Geometry: final body of the model. Coordinates: model frame, mm. Face numbers are marked on the shaded views. A direction names the side the tool comes from. Round coordinates to 2 decimals unless told otherwise and drop trailing zeros. Loops run counter-clockwise (first coordinate to the right, second up) from the corner with the lowest first, then second, coordinate; pieces in that order, holes last. Notation, with made-up numbers: (67.25, 9.25) - (76.25, 9.25) arc R13 ccw to (76.25, 21.25) - close; hole circle Ø9 at (80, -9.5). An arc over 180 degrees is marked (long way). Write item = value, one per line. Start each with the question number.
Item 1: Draft query along Y for the marked faces 4, 5 and 6. Return one class per face: pulls with the +Y half, pulls with the -Y half, needs draft (parallel to the pull), parting line crosses it, or undercut.
Item 2: First-contact query: pin 1 (1.5 mm diameter, centred on x = 8, y = 0, fed in from -Z); pin 2 (0.7 mm diameter, centred on x = 0.5, z = 0.5, fed in from -Y). Flat tips, straight axial feed; report the tip coordinate or a pass-through.
Item 3: Line query: line 1 (X direction, y = 1, z = -3.5); line 2 (Y direction, x = 1, z = 0.75); line 3 (Z direction, x = 17.25, y = 1.5). Output: solid intervals per line, ascending. Write a range as from..to.
Item 4: Access query for the marked faces 1, 2 and 3. Directions: +Z, -Z, +X, -X, +Y, -Y. A direction counts if a zero-diameter tool reaches every point of the face in a straight line with its end or side. Return the directions, or none.
Item 5: Section A-A (x = 15). Return loops of the section in (y, z).
from build123d import *

# Parameters (mm, degrees)
SKETCH1_R           = 4.25
BASEHEAD_DEPTH      = 5
SKETCH2_R           = 2.5
BASEBODY_DEPTH      = 16
HEXAGONSOCKET_DEPTH = 2.5
TOPFILLET_R         = 0.625
CHAMFER1_SIZE       = 0.2


with BuildPart() as part:
    # Sketch1 → BaseHead (new body)
    with BuildSketch(Plane(origin=(0, 0, 0), x_dir=(0, 0, -1), z_dir=(1, 0, 0))):
        Circle(SKETCH1_R)
    extrude(amount=BASEHEAD_DEPTH)

    # Sketch2 → BaseBody (add)
    with BuildSketch(Plane(origin=(5, 0, 0), x_dir=(0, 0, -1), z_dir=(1, 0, 0))):
        Circle(SKETCH2_R)
    extrude(amount=BASEBODY_DEPTH)

    # Sketch3 → HexagonSocket (cut)
    with BuildSketch(Plane(origin=(0, 0, 0), x_dir=(0, 0, -1), z_dir=(1, 0, 0))):
        Polygon((2.309401077, 0), (1.154700538, 2), (-1.154700538, 2), (-2.309401077, 0), (-1.154700538, -2), (1.154700538, -2), align=None)
    extrude(amount=HEXAGONSOCKET_DEPTH, mode=Mode.SUBTRACT)

    # Sketch4 → Cut-Revolve1 (revolve, cut)
    with BuildSketch(Plane(origin=(-4.19613823, 0.75, 0), x_dir=(-1, 0, 0), z_dir=(0, 0, 1))):
        Polygon((-6.69613823, 2.75), (-7.850838768, 0.75), (-6.69613823, 0.75), align=None)
    revolve(axis=Axis((0.838992387, 0, 0), (-1, 0, 0)), mode=Mode.SUBTRACT)

    # TopFillet
    topfillet_edges = [part.edges().sort_by_distance(p)[0] for p in [
        (0, 0, 4.25),
    ]]
    fillet(topfillet_edges, radius=TOPFILLET_R)

    # Chamfer1
    chamfer1_edges = [part.edges().sort_by_distance(p)[0] for p in [
        (21, 0, 2.5),
    ]]
    chamfer(chamfer1_edges, length=CHAMFER1_SIZE)


solid = part.part
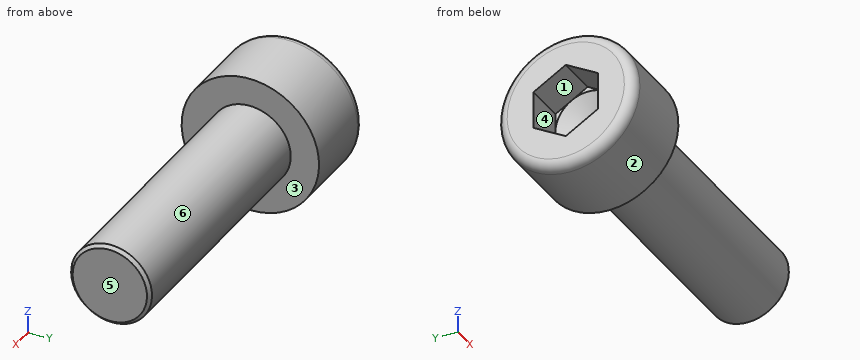
Taken from the geometry:
q1.face_4 = undercut
q1.face_5 = needs draft
q1.face_6 = parting line crosses it
q2.pin_1 = -2.5
q2.pin_2 = -4.25
q3.line_1 = 0..5
q3.line_2 = -4.18..-2, 2..4.18
q3.line_3 = -2..2
q4.face_1 = -X
q4.face_2 = +X, -X
q4.face_3 = +X
q5.outline = circle Ø5 at (0, 0)
